```python
from build123d import *

# Parameters (mm, degrees)
SKETCH_1_R          = 2
EXTRUDE_1_DEPTH     = 2
SKETCH_4_W          = 8
SKETCH_4_H          = 2
EXTRUDE_3_DEPTH     = 35.5
SKETCH_5_R          = 1
CUT_EXTRUDE_1_DEPTH = 8
SKETCH_6_W          = 8
SKETCH_6_H          = 10
EXTRUDE_4_DEPTH     = 2
SKETCH_7_R          = 2
CUT_EXTRUDE_2_DEPTH = 2
EXTRUDE_5_DEPTH     = 4.5
EXTRUDE_6_DEPTH     = 4.5
FILLET_1_R          = 3
SKETCH_10_W         = 17
SKETCH_10_H         = 24
SKETCH_10_R         = 1
SKETCH_10_R_2       = 2
EXTRUDE_7_DEPTH     = 1
SKETCH_12_W         = 17
SKETCH_12_H         = 35.5
EXTRUDE_8_DEPTH     = 0.5
SKETCH_13_W         = 17
SKETCH_13_H         = 35.5
EXTRUDE_9_DEPTH     = 0.5
EXTRUDE_START       = 1
SKETCH_14_R         = 2
EXTRUDE_10_DEPTH    = 1
SKETCH_16_W         = 17
SKETCH_16_H         = 35.5
EXTRUDE_11_DEPTH    = 0.5
SKETCH_17_W         = 17
SKETCH_17_H         = 35.5
EXTRUDE_12_DEPTH    = 0.5
EXTRUDE_START_2     = -3
SKETCH_18_R         = 1
EXTRUDE_13_DEPTH    = 3
SKETCH_19_R         = 5
CUT_EXTRUDE_3_DEPTH = 3
SKETCH_20_W         = 8
SKETCH_20_H         = 20
CUT_EXTRUDE_4_DEPTH = 34
FILLET_3_R          = 2
FILLET_4_R          = 3


with BuildPart() as part:
    # 草图1 → 凸台-拉伸1 (new body)
    # profile 1 of 5: a face of its own
    with BuildSketch(Plane.XY):
        with BuildLine():
            Line((4, 6.34428877), (4, -6.34428877))
            ThreePointArc((4, -6.34428877), (6.566962768, -3.622844187), (7.5, 0))
            ThreePointArc((7.5, 0), (6.566962768, 3.622844187), (4, 6.34428877))
        make_face()
    # profile 2 of 5: a face of its own
    with BuildSketch(Plane.XY):
        with BuildLine():
            Line((-4, 6.34428877), (-4, -6.34428877))
            ThreePointArc((-4, -6.34428877), (0, -7.5), (4, -6.34428877))
            Line((4, -6.34428877), (4, 6.34428877))
            ThreePointArc((4, 6.34428877), (0, 7.5), (-4, 6.34428877))
        make_face()
        Circle(SKETCH_1_R, mode=Mode.SUBTRACT)
    # profile 3 of 5: a face of its own
    with BuildSketch(Plane.XY):
        with BuildLine():
            ThreePointArc((-4, 6.34428877), (-7.5, 0), (-4, -6.34428877))
            Line((-4, -6.34428877), (-4, 6.34428877))
        make_face()
    # profile 4 of 5: a face of its own
    with BuildSketch(Plane.XY):
        with BuildLine():
            Line((-4, 10), (-4, 6.34428877))
            ThreePointArc((-4, 6.34428877), (0, 7.5), (4, 6.34428877))
            Line((4, 6.34428877), (4, 10))
            Line((4, 10), (-4, 10))
        make_face()
    # profile 5 of 5: a face of its own
    with BuildSketch(Plane.XY):
        with BuildLine():
            Line((-4, -6.34428877), (-4, -10))
            Line((-4, -10), (4, -10))
            Line((4, -10), (4, -6.34428877))
            ThreePointArc((4, -6.34428877), (0, -7.5), (-4, -6.34428877))
        make_face()
    extrude(amount=EXTRUDE_1_DEPTH)

    # 草图4 → 凸台-拉伸3 (add)
    with BuildSketch(Plane.XY.offset(2)):
        with Locations((0, -11)):
            Rectangle(SKETCH_4_W, SKETCH_4_H)
        with Locations((0, 11)):
            Rectangle(SKETCH_4_W, SKETCH_4_H)
    extrude(amount=-EXTRUDE_3_DEPTH)

    # 草图5 → 切除-拉伸1 (cut)
    with BuildSketch(Plane(origin=(0, 0, 0), x_dir=(-1, 0, 0), z_dir=(0, 0, -1))):
        with Locations((0, 5.5)):
            Circle(SKETCH_5_R)
        with Locations((0, -5.5)):
            Circle(SKETCH_5_R)
    extrude(amount=-CUT_EXTRUDE_1_DEPTH, mode=Mode.SUBTRACT)

    # 草图6 → 凸台-拉伸4 (add)
    with BuildSketch(Plane(origin=(0, 0, -33.5), x_dir=(-1, 0, 0), z_dir=(0, 0, -1))):
        with Locations((0, -15)):
            Rectangle(SKETCH_6_W, SKETCH_6_H)
        with Locations((0, 15)):
            Rectangle(SKETCH_6_W, SKETCH_6_H)
    extrude(amount=EXTRUDE_4_DEPTH)

    # 草图7 → 切除-拉伸2 (cut)
    with BuildSketch(Plane.XY.offset(-33.5)):
        with Locations((0, 16)):
            Circle(SKETCH_7_R)
        with Locations((0, -16)):
            Circle(SKETCH_7_R)
    extrude(amount=-CUT_EXTRUDE_2_DEPTH, mode=Mode.SUBTRACT)

    # 草图8 → 凸台-拉伸5 (add)
    with BuildSketch(Plane.ZY.offset(4)):
        Polygon((-35.5, 10), (0, 10), (0, 6.34428877), (2, 6.34428877), (2, 12), (-33.5, 12), (-33.5, 20), (-35.5, 20), align=None)
        Polygon((-33.5, -12), (2, -12), (2, -6.34428877), (2, 6.34428877), (0, 6.34428877), (0, -6.34428877), (0, -10), (-35.5, -10), (-35.5, -20), (-33.5, -20), align=None)
    extrude(amount=EXTRUDE_5_DEPTH)

    # 草图9 → 凸台-拉伸6 (add)
    with BuildSketch(Plane(origin=(4, 0, 0), x_dir=(0, 0, -1), z_dir=(1, 0, 0))):
        Polygon((-2, 6.34428877), (-2, -6.34428877), (-2, -12), (33.5, -12), (33.5, -20), (35.5, -20), (35.5, -10), (0, -10), (0, -6.34428877), (0, 6.34428877), (0, 10), (35.5, 10), (35.5, 20), (33.5, 20), (33.5, 12), (-2, 12), align=None)
    extrude(amount=EXTRUDE_6_DEPTH)

    # 圆角1
    fillet_1_edges = [part.edges().sort_by_distance(p)[0] for p in [
        (-8.5, -20, -34.5),
        (-8.5, 20, -34.5),
        (8.5, 20, -34.5),
        (8.5, -20, -34.5),
    ]]
    fillet(fillet_1_edges, radius=FILLET_1_R)

    # 草图10 → 凸台-拉伸7 (add)
    with BuildSketch(Plane.XY.offset(2)):
        Rectangle(SKETCH_10_W, SKETCH_10_H)
        with Locations(Location((0, -5.5, 0), (0, 0, 180))):
            Circle(SKETCH_10_R, mode=Mode.SUBTRACT)
        Circle(SKETCH_10_R_2, mode=Mode.SUBTRACT)
        with Locations(Location((0, 5.5, 0), (0, 0, 180))):
            Circle(SKETCH_10_R, mode=Mode.SUBTRACT)
    extrude(amount=EXTRUDE_7_DEPTH)

    # 草图12 → 凸台-拉伸8 (add)
    with BuildSketch(Plane.XZ.offset(-10)):
        with Locations((0, -17.75)):
            Rectangle(SKETCH_12_W, SKETCH_12_H)
    extrude(amount=EXTRUDE_8_DEPTH)

    # 草图13 → 凸台-拉伸9 (add)
    with BuildSketch(Plane(origin=(0, -10, 0), x_dir=(1, 0, 0), z_dir=(0, 1, 0))):
        with Locations((0, 17.75)):
            Rectangle(SKETCH_13_W, SKETCH_13_H)
    extrude(amount=EXTRUDE_9_DEPTH)

    # 草图14 → 凸台-拉伸10 (add)
    # profile 1 of 2: a face of its own
    with BuildSketch(Plane.XY.offset(-33.5).offset(EXTRUDE_START)):
        with BuildLine():
            Line((-8.5, -12), (-8.5, -17))
            ThreePointArc((-8.5, -17), (-7.621320344, -19.121320344), (-5.5, -20))
            Line((-5.5, -20), (5.5, -20))
            ThreePointArc((5.5, -20), (7.621320344, -19.121320344), (8.5, -17))
            Line((8.5, -17), (8.5, -12))
            Line((8.5, -12), (-8.5, -12))
        make_face()
        with Locations((0, -16)):
            Circle(SKETCH_14_R, mode=Mode.SUBTRACT)
    # profile 2 of 2: a face of its own
    with BuildSketch(Plane.XY.offset(-33.5).offset(EXTRUDE_START)):
        with BuildLine():
            Line((5.5, 20), (-5.5, 20))
            ThreePointArc((-5.5, 20), (-7.621320344, 19.121320344), (-8.5, 17))
            Line((-8.5, 17), (-8.5, 12))
            Line((-8.5, 12), (8.5, 12))
            Line((8.5, 12), (8.5, 17))
            ThreePointArc((8.5, 17), (7.621320344, 19.121320344), (5.5, 20))
        make_face()
        with Locations((0, 16)):
            Circle(SKETCH_14_R, mode=Mode.SUBTRACT)
    extrude(amount=-EXTRUDE_10_DEPTH)

    # 草图16 → 凸台-拉伸11 (add)
    with BuildSketch(Plane.XZ.offset(12)):
        with Locations((0, -14.75)):
            Rectangle(SKETCH_16_W, SKETCH_16_H)
    extrude(amount=EXTRUDE_11_DEPTH)

    # 草图17 → 凸台-拉伸12 (add)
    with BuildSketch(Plane(origin=(0, 12, 0), x_dir=(1, 0, 0), z_dir=(0, 1, 0))):
        with Locations((0, 14.75)):
            Rectangle(SKETCH_17_W, SKETCH_17_H)
    extrude(amount=EXTRUDE_12_DEPTH)

    # 草图18 → 凸台-拉伸13 (add)
    with BuildSketch(Plane.XY.offset(3).offset(EXTRUDE_START_2)):
        with Locations((0, -5.5)):
            Circle(SKETCH_18_R)
        with Locations((0, 5.5)):
            Circle(SKETCH_18_R)
    extrude(amount=EXTRUDE_13_DEPTH)

    # 草图19 → 切除-拉伸3 (cut)
    with BuildSketch(Plane.XY.offset(3)):
        Circle(SKETCH_19_R)
    extrude(amount=-CUT_EXTRUDE_3_DEPTH, mode=Mode.SUBTRACT)

    # 草图20 → 切除-拉伸4 (cut)
    with BuildSketch(Plane(origin=(0, 12.5, 0), x_dir=(1, 0, 0), z_dir=(0, 1, 0))):
        with Locations((0, 16.249764914)):
            Rectangle(SKETCH_20_W, SKETCH_20_H)
    extrude(amount=-CUT_EXTRUDE_4_DEPTH, mode=Mode.SUBTRACT)

    # 圆角3
    fillet_3_edges = [part.edges().sort_by_distance(p)[0] for p in [
        (4, 11, -26.249764914),
        (4, 11, -6.249764914),
        (-4, 11, -6.249764914),
        (-4, 11, -26.249764914),
        (4, -11, -26.249764914),
        (4, -11, -6.249764914),
        (-4, -11, -6.249764914),
        (-4, -11, -26.249764914),
    ]]
    fillet(fillet_3_edges, radius=FILLET_3_R)

    # 圆角4
    fillet_4_edges = [part.edges().sort_by_distance(p)[0] for p in [
        (0, -12.5, 3),
        (0, 12.5, 3),
    ]]
    fillet(fillet_4_edges, radius=FILLET_4_R)


solid = part.part
```
Work out the finished part from the listing and answer in its coordinate system (mm). A direction names the side the tool comes from. Give positions to 0.01 mm unless a question says otherwise; leave off trailing zeros. Order: outer loops, then holes, each group sorted by start corner. A loop starts at its lowest first (then second) coordinate and runs counter-clockwise, first axis right, second up.
1. For faces 1 (the flat face through (-2, 15, -32.5)), 2 (the flat face through (-4, -11, -16)), 3 (the cylindrical face through (0.12, -11.64, 2.1)), determine the directions among +Z, -Z, +X, -X, +Y, -Y from which every point of the face is accessible in a straight line to the end or side of a thin tool.
Result sheet:
face 1: +Z, +X, -X, +Y
face 2: +Y, -Y
face 3: +Z, +X, -X, -Y
2. Section A-A, the plane y = 16 is taken. Determine the outline of the cut face in (x, z), and give its area (3 significant figures).
Result sheet:
outline: (-8.5, -35.5) - (-2, -35.5) - (-2, -32.5) - (-8.5, -32.5) - close; (2, -35.5) - (8.5, -35.5) - (8.5, -32.5) - (2, -32.5) - close
area: 39.0 mm2
3. Section C-C, the plane z = -27.5 is taken. Determine the outline of the cut face in (x, y), and give its area (3 significant figures).
Result sheet:
outline: (-8.5, -12.5) - (8.5, -12.5) - (8.5, -9.5) - (-8.5, -9.5) - close; (-8.5, 9.5) - (8.5, 9.5) - (8.5, 12.5) - (-8.5, 12.5) - close
area: 102 mm2
4. The mould has two halves that part along Y. Classify faces 4 (the cylindrical face through (0, -14, -34)), 5 (the flat face through (0, -20, -34)), 6 (the flat face through (-6, 9.5, -18)), 7 (the cylindrical face through (3.43, 10.98, -6.85)): released by +Y, released by -Y, zero draft, split by the parting line, or undercut.
Result sheet:
face 4: undercut
face 5: released by -Y
face 6: undercut
face 7: zero draft
5. Straight lines are drawn through the part: L1, parallel to Y at x = 0, z = -33.6; L2, parallel to Y at x = -4.5, z = -30.5; L3, parallel to X at y = -11.5, z = -15. For each, find the intervals that lie inside material, in ascending order.
Result sheet:
L1: y = -20 to -18, -14 to -9.5, 9.5 to 14, 18 to 20
L2: y = -12.5 to -9.5, 9.5 to 12.5
L3: x = -8.5 to -4, 4 to 8.5
6. Each of these flat-tipped pins is pushed along its axis until it touches: P1, Ø1.5, axis at x = -3.5, z = -26.5, coming from the -Y side; P2, Ø10, axis at x = -2, y = -2, coming from the -Z side; P3, Ø10, axis at x = 0.5, y = 13, coming from the +Z side; P4, Ø8, axis at x = 0.5, y = 17.5, coming from the +Z side. Where does it stop, or does it pass through?
Result sheet:
P1: stops at y = -12.5
P2: stops at z = 0
P3: stops at z = 3
P4: stops at z = -32.5
7. Section D-D, the plane z = -10.5 is taken. Determine the outline of the cut face in (x, y), and give its area (3 significant figures).
Result sheet:
outline: (-8.5, -12.5) - (-4, -12.5) - (-4, -9.5) - (-8.5, -9.5) - close; (-8.5, 9.5) - (-4, 9.5) - (-4, 12.5) - (-8.5, 12.5) - close; (4, -12.5) - (8.5, -12.5) - (8.5, -9.5) - (4, -9.5) - close; (4, 9.5) - (8.5, 9.5) - (8.5, 12.5) - (4, 12.5) - close
area: 54.0 mm2
8. Section B-B, the plane x = 0 is taken. Give the number of separate pieces and of enclosed holes in the cut face, and give its area (3 significant figures).
Result sheet:
separate pieces: 6
enclosed holes: 0
area: 155 mm2
